from build123d import *

# Parameters (mm, degrees)
F0_W     = 74.433348
F0_H     = 67.411334
F1_DEPTH = 25.4
F2_R     = 10.968737
F3_DEPTH = 25.401
F4_R     = 7.851637
F5_DEPTH = 76.2


with BuildPart() as f1:
    # F0 (on Top) → F1 (new body)
    with BuildSketch(Plane.XY):
        with Locations((1e-06, 4e-06)):
            Rectangle(F0_W, F0_H)
    extrude(amount=F1_DEPTH)

    # F2 (on face) → F3 (cut, through all)
    with BuildSketch(Plane.XY.offset(25.4)):
        Circle(F2_R)
    extrude(amount=-F3_DEPTH, mode=Mode.SUBTRACT)

    # F4 (on face) → F5 (join)
    with BuildSketch(Plane.XY.offset(25.4)):
        with Locations((-27.759731, 23.318172)):
            Circle(F4_R)
    extrude(amount=F5_DEPTH)


solid = f1.part
Source: CAD feature listing. Evaluate the final solid. Frame: model axes, mm. A direction names the side the tool comes from. Coordinates: 2 decimals unless noted, no trailing zeros. Loops run counter-clockwise (first coordinate to the right, second up) from the corner with the lowest first, then second, coordinate; pieces in that order, holes last. Notation, with made-up numbers: (81.5, -6) - (96.5, -6) arc R25 ccw to (96.5, 6) - close; hole circle Ø1 at (-39, 7). An arc over 180 degrees is marked (long way). One line per item, written item: value. Start each with the question number.
1. Section A-A (y = 0). Return the cut outline in (x, z), and give its area (3 significant figures).
2. Mould query, pull axis Y, two halves, no side actions, for faces 1 (the cylindrical face through (-2.378, -10.708, 12.878)), 2 (the flat face through (-37.217, 0, 13)), 3 (the flat face through (-1, -33.706, 13)). Classes: pulls with the +Y half, pulls with the -Y half, needs draft (parallel to the pull), parting line crosses it, or undercut.
3. Section D-D (y = 19). Return the cut outline in (x, z), and give its area (3 significant figures).
4. Section C-C (x = -30). Return the cut outline in (y, z).
5. Ray query, L1, parallel to Y at x = 0, z = 16; L2, parallel to Z at x = -19.5, y = -21.5; L3, parallel to Y at x = -32, z = 43.5. Return the intervals inside material, ascending.
6. Section B-B (x = 0). Return the cut outline in (y, z).
7. Contact query for flat-ended pins moving along their axis: P1, Ø1.5, axis at x = -11, y = 7.5, coming from the +Z side; P2, Ø2, axis at y = 26, z = 45, coming from the +X side. Output: stop coordinate, or through.
8. Set-up query: faces 4 (the flat face through (-1, 33.706, 13)), 5 (the cylindrical face through (-29.462, 15.653, 62.967)). Return all of +Z, -Z, +X, -X, +Y, -Y with unobstructed straight access to the full face (end or side cutting, diameter ignored); none if empty.
Verdict:
1. outline: (-37.22, 0) - (-10.97, 0) - (-10.97, 25.4) - (-37.22, 25.4) - close; (10.97, 0) - (37.22, 0) - (37.22, 25.4) - (10.97, 25.4) - close
1. area: 1,330 mm2
2. face 1: undercut
2. face 2: needs draft
2. face 3: pulls with the -Y half
3. outline: (-37.22, 0) - (37.22, 0) - (37.22, 25.4) - (-21.2, 25.4) - (-21.2, 101.6) - (-34.32, 101.6) - (-34.32, 25.4) - (-37.22, 25.4) - close
3. area: 2,890 mm2
4. outline: (-33.71, 0) - (33.71, 0) - (33.71, 25.4) - (30.84, 25.4) - (30.84, 101.6) - (15.79, 101.6) - (15.79, 25.4) - (-33.71, 25.4) - close
5. L1: y = -33.71 to -10.97, 10.97 to 33.71
5. L2: z = 0 to 25.4
5. L3: y = 16.71 to 29.93
6. outline: (-33.71, 0) - (-10.97, 0) - (-10.97, 25.4) - (-33.71, 25.4) - close; (10.97, 0) - (33.71, 0) - (33.71, 25.4) - (10.97, 25.4) - close
7. P1: stops at z = 25.4
7. P2: stops at x = -20.09
8. face 4: +Z, -Z, +X, -X, +Y
8. face 5: +Z
